Work out the finished part from the listing and answer in its coordinate system (mm). Coordinates: 2 decimals unless noted, no trailing zeros. Order: outer loops, then holes, each group sorted by start corner. A loop starts at its lowest first (then second) coordinate and runs counter-clockwise, first axis right, second up. Notation, with made-up numbers: M -30,-16 L 21,-16 A20 cw 21,-11 Z; hole C -34,16 d8. An arc over 180 degrees is marked long. Use a Markdown table: item, result.
from build123d import *

# Parameters (mm, degrees)
SKETCH1_W               = 25.4
SKETCH1_H               = 2.7432
BOSS_EXTRUDE1_DEPTH     = 203.2
CUT_EXTRUDE1_DEPTH      = 111.720339735
CUT_EXTRUDE1_DEPTH_BACK = 111.720339735
SKETCH2_R               = 3.96875


with BuildPart() as part:
    # Sketch1 → Boss-Extrude1 (new body)
    with BuildSketch(Plane(origin=(0, 0, 0), x_dir=(1, 0, 0), z_dir=(0, 1, 0))):
        with Locations((12.7, -1.3716)):
            Rectangle(SKETCH1_W, SKETCH1_H)
    extrude(amount=BOSS_EXTRUDE1_DEPTH)

    # Sketch2 → Cut-Extrude1 (cut, two sides: drawn at the far end of the back side and taken through both)
    with BuildSketch(Plane(origin=(-3.908296933, 106.606717755, 5.9182), x_dir=(1, 0, 0), z_dir=(0, 0, 1)).offset(-CUT_EXTRUDE1_DEPTH_BACK)):
        with Locations((3.908296933, 64.843282245)):
            Circle(SKETCH2_R)
        with Locations((3.908296933, -74.856717755)):
            Circle(SKETCH2_R)
    extrude(amount=CUT_EXTRUDE1_DEPTH + CUT_EXTRUDE1_DEPTH_BACK, mode=Mode.SUBTRACT)


solid = part.part
(1) A cutting plane is placed at A-A (y = 171.45). Determine the outline of the cut face in (x, z), then the cut area to 3 significant figures.
Conclusion:
| item | result |
|---|---|
| outline | M 3.97,0 L 25.4,0 L 25.4,2.74 L 3.97,2.74 Z |
| area | 58.8 mm2 |
(2) Determine the mould class of faces 1 (the cylindrical face through (3.968, 31.663, 1.352)), 2 (the flat face through (13, 100, 0)) for opening direction Y: pulls with the +Y half, pulls with the -Y half, needs draft (parallel to the pull), parting line crosses it, or undercut.
Conclusion:
| item | result |
|---|---|
| face 1 | undercut |
| face 2 | needs draft |
(3) Straight lines are drawn through the part: L1, parallel to Y at x = 2.5, z = 0.9; L2, parallel to Y at x = 3, z = 0.4; L3, parallel to X at y = 169.5, z = 1.4. For each, find the intervals that lie inside material, in ascending order.
Conclusion:
| item | result |
|---|---|
| L1 | 0 to 28.67, 34.83 to 168.37, 174.53 to 203.2 |
| L2 | 0 to 29.15, 34.35 to 168.85, 174.05 to 203.2 |
| L3 | 3.46 to 25.4 |
